Geometry: final body of the model. Coordinates: model frame, mm. A direction names the side the tool comes from. Give positions to 0.01 mm unless a question says otherwise; leave off trailing zeros. Write each loop counter-clockwise with the first axis right and the second up, starting at its lowest first coordinate (ties: lowest second). Pieces come first, ordered by that corner, then holes. Notation, with made-up numbers: (74, 89) -> (133, 89) arc R25 cw to (133, 106) -> close; hole circle Ø5 at (31.25, -37.5). An arc over 180 degrees is marked (long way). Answer as a JSON object with one key per item and string values. Group by question number.
(1) Contact query for flat-ended pins moving along their axis: pin 1 Ø3 at (x, y) = (10, -12.5) entering from +Z; pin 2 Ø5 at (x, z) = (0, 8.5) entering from +Y; pin 3 Ø2 at (x, y) = (12, -38) entering from -Z. Output: stop coordinate, or through.
(2) Set-up query: faces 4 (the face through (-5.89, -30.65, 2.86)), 5 (the face through (-0.28, 38.6, 0.86)), 6 (the face through (16.25, -38.51, 5.96)), 7 (the face through (16.75, -35.53, 6.05)). Return all of +Z, -Z, +X, -X, +Y, -Y with unobstructed straight access to the full face (end or side cutting, diameter ignored); none if empty.
(3) Material intervals for probe 1 along Y at (x, z) = (-10.5, 11.5); probe 2 along X at (y, z) = (3.5, 4.5); probe 3 along X at (y, z) = (9, 11.5), sorted ascending.
(4) Draft query along Z for faces 1 (the face through (24.196, -36.789, 13.507)), 2 (the face through (0.28, -38.6, 0.86)), 3 (the face through (11, -39, 4.25)). Return one class per face: +Z half, -Z half, draft (parallel to the pull), parting line (faces both ways), or undercut.
(5) Section query C-C on y = 27. Output: boundary loops of the cut face in (x, z).
(6) Section query B-B on y = -4.5. Output: boundary loops of the cut face in (x, z).
(7) Section query A-A on x = -10. Output: boundary loops of the cut face in (y, z).
from build123d import *

# Parameters (mm, degrees)
PAD_DEPTH       = 2
PAD001_DEPTH    = 12
FILLET_R        = 3
SKETCH002_R     = 2
POCKET_DEPTH    = 5
POCKET003_DEPTH = 1
SKETCH016_W     = 16
SKETCH016_H     = 2
PAD007_DEPTH    = 10
FILLET002_R     = 3
PAD008_DEPTH    = 4
SKETCH019_R     = 3.25
POCKET005_DEPTH = 2
FILLET004_R     = 1
SKETCH020_W     = 5
SKETCH020_H     = 50
PAD009_DEPTH    = 8
FILLET005_R     = 2
SKETCH021_R     = 3.25
POCKET006_DEPTH = 50


with BuildPart() as part:
    # Sketch → Pad (new body)
    with BuildSketch(Plane.XY):
        with BuildLine():
            Line((-27, 32.5), (-27, -32.5))
            ThreePointArc((-27, -32.5), (-24.949747, -37.449747), (-20, -39.5))
            Line((-20, -39.5), (20, -39.5))
            ThreePointArc((20, -39.5), (24.949747, -37.449747), (27, -32.5))
            Line((27, -32.5), (27, 32.5))
            ThreePointArc((27, 32.5), (24.949747, 37.449747), (20, 39.5))
            Line((20, 39.5), (-20, 39.5))
            ThreePointArc((-20, 39.5), (-24.949747, 37.449747), (-27, 32.5))
        make_face()
    extrude(amount=PAD_DEPTH)

    # Sketch001 (on Face10 of Pad) → Pad001 (join)
    with BuildSketch(Plane.XY.offset(2)):
        with BuildLine():
            Line((-27, 32.5), (-27, -32.5))
            ThreePointArc((-27, -32.5), (-24.949747, -37.449747), (-20, -39.5))
            Line((-20, -39.5), (20, -39.5))
            ThreePointArc((20, -39.5), (24.949747, -37.449747), (27, -32.5))
            Line((27, -32.5), (27, 32.5))
            ThreePointArc((27, 32.5), (24.949747, 37.449747), (20, 39.5))
            Line((20, 39.5), (-20, 39.5))
            ThreePointArc((-20, 39.5), (-24.949747, 37.449747), (-27, 32.5))
        make_face()
        with BuildLine():
            Line((-25, 32.5), (-25, -32.5))
            ThreePointArc((-25, -32.5), (-23.535534, -36.035534), (-20, -37.5))
            Line((-20, -37.5), (20, -37.5))
            ThreePointArc((20, -37.5), (23.535534, -36.035534), (25, -32.5))
            Line((25, -32.5), (25, 32.5))
            ThreePointArc((25, 32.5), (23.535534, 36.035534), (20, 37.5))
            Line((20, 37.5), (-20, 37.5))
            ThreePointArc((-20, 37.5), (-23.535534, 36.035534), (-25, 32.5))
        make_face(mode=Mode.SUBTRACT)
    extrude(amount=PAD001_DEPTH)

    # Fillet
    fillet_edges = [part.edges().sort_by_distance(p)[0] for p in [
        (0, -39.5, 0),
    ]]
    fillet(fillet_edges, radius=FILLET_R)

    # Sketch002 (on Face10 of Fillet) → Pocket (cut)
    with BuildSketch(Plane.XZ.offset(39.5)):
        with Locations((-10, 8.5)):
            Circle(SKETCH002_R)
        with BuildLine():
            ThreePointArc((8.3, 7.75), (6.55, 6), (8.3, 4.25))
            Line((8.3, 4.25), (14.5, 4.25))
            ThreePointArc((14.5, 4.25), (16.25, 6), (14.5, 7.75))
            Line((8.3, 7.75), (14.5, 7.75))
        make_face()
    extrude(amount=-POCKET_DEPTH, mode=Mode.SUBTRACT)

    # Sketch007 → Pocket003 (cut)
    with BuildSketch(Plane.XY.offset(14)):
        with BuildLine():
            Line((-26, 32.5), (-26, -32.5))
            ThreePointArc((-26, -32.5), (-24.242641, -36.742641), (-20, -38.5))
            Line((-20, -38.5), (20, -38.5))
            ThreePointArc((20, -38.5), (24.242641, -36.742641), (26, -32.5))
            Line((26, -32.5), (26, 32.5))
            ThreePointArc((26, 32.5), (24.242641, 36.742641), (20, 38.5))
            Line((20, 38.5), (-20, 38.5))
            ThreePointArc((-20, 38.5), (-24.242641, 36.742641), (-26, 32.5))
        make_face()
        with BuildLine():
            Line((-25, 32.5), (-25, -32.5))
            ThreePointArc((-25, -32.5), (-23.535534, -36.035534), (-20, -37.5))
            Line((-20, -37.5), (20, -37.5))
            ThreePointArc((20, -37.5), (23.535534, -36.035534), (25, -32.5))
            Line((25, -32.5), (25, 32.5))
            ThreePointArc((25, 32.5), (23.535534, 36.035534), (20, 37.5))
            Line((20, 37.5), (-20, 37.5))
            ThreePointArc((-20, 37.5), (-23.535534, 36.035534), (-25, 32.5))
        make_face(mode=Mode.SUBTRACT)
    extrude(amount=-POCKET003_DEPTH, mode=Mode.SUBTRACT)

    # Sketch016 (on Face34 of Pocket003) → Pad007 (join)
    with BuildSketch(Plane.XY.offset(2)):
        with Locations((-6, -32.55)):
            Rectangle(SKETCH016_W, SKETCH016_H)
    extrude(amount=PAD007_DEPTH)

    # Fillet002
    fillet002_edges = [part.edges().sort_by_distance(p)[0] for p in [
        (-6, -31.55, 2),
    ]]
    fillet(fillet002_edges, radius=FILLET002_R)

    # Sketch017 (on Face12 of Fillet002) → Pad008 (join)
    with BuildSketch(Plane(origin=(0, -37.5, 0), x_dir=(-1, 0, 0), z_dir=(0, 1, 0))):
        with BuildLine():
            ThreePointArc((-14.5, 8.25), (-16.75, 6), (-14.5, 3.75))
            Line((-14.5, 3.75), (-8.3, 3.75))
            ThreePointArc((-8.3, 3.75), (-6.05, 6), (-8.3, 8.25))
            Line((-14.5, 8.25), (-8.3, 8.25))
        make_face()
        with BuildLine():
            ThreePointArc((-14.5, 7.85), (-16.35, 6), (-14.5, 4.15))
            Line((-14.5, 4.15), (-8.3, 4.15))
            ThreePointArc((-8.3, 4.15), (-6.45, 6), (-8.3, 7.85))
            Line((-14.5, 7.85), (-8.3, 7.85))
        make_face(mode=Mode.SUBTRACT)
    extrude(amount=PAD008_DEPTH)

    # Sketch019 (on Face46 of Pad008) → Pocket005 (cut)
    with BuildSketch(Plane(origin=(0, 39.5, 0), x_dir=(-1, 0, 0), z_dir=(0, 1, 0))):
        with Locations((0, 8.5)):
            Circle(SKETCH019_R)
    extrude(amount=-POCKET005_DEPTH, mode=Mode.SUBTRACT)

    # Fillet004
    fillet004_edges = [part.edges().sort_by_distance(p)[0] for p in [
        (3.25, 39.5, 8.5),
    ]]
    fillet(fillet004_edges, radius=FILLET004_R)

    # Sketch020 (on Face5 of Fillet004) → Pad009 (join)
    with BuildSketch(Plane.XY.offset(2)):
        Rectangle(SKETCH020_W, SKETCH020_H)
    extrude(amount=PAD009_DEPTH)

    # Fillet005
    fillet005_edges = [part.edges().sort_by_distance(p)[0] for p in [
        (2.5, 0, 2),
        (-2.5, 0, 2),
    ]]
    fillet(fillet005_edges, radius=FILLET005_R)

    # Sketch021 (on Face4 of Fillet005) → Pocket006 (cut)
    with BuildSketch(Plane(origin=(0, 25, 0), x_dir=(-1, 0, 0), z_dir=(0, 1, 0))):
        with Locations((0, 8.5)):
            Circle(SKETCH021_R)
    extrude(amount=-POCKET006_DEPTH, mode=Mode.SUBTRACT)


solid = part.part
Answer list:
{
 "1": {"pin 1": "z = 2", "pin 2": "y = -31.55", "pin 3": "z = 0.04"},
 "2": {"face 4": "+Z", "face 5": "-Z, +X, -X, +Y", "face 6": "-Y", "face 7": "none"},
 "3": {"probe 1": "-39.5 to -37.5, -33.55 to -31.55, 37.5 to 39.5", "probe 2": "-27 to -25, -2.5 to 2.5, 25 to 27", "probe 3": "-27 to -25, 25 to 27"},
 "4": {"face 1": "draft", "face 2": "-Z half", "face 3": "undercut"},
 "5": {"outline": "(-27, 3) arc R3 ccw to (-24, 0) -> (24, 0) arc R3 ccw to (27, 3) -> (27, 14) -> (26, 14) -> (26, 13) -> (25, 13) -> (25, 2) -> (-25, 2) -> (-25, 13) -> (-26, 13) -> (-26, 14) -> (-27, 14) -> close"},
 "6": {"outline": "(-27, 3) arc R3 ccw to (-24, 0) -> (24, 0) arc R3 ccw to (27, 3) -> (27, 14) -> (26, 14) -> (26, 13) -> (25, 13) -> (25, 2) -> (4.5, 2) arc R2 cw to (2.5, 4) -> (2.5, 6.42) arc R3.25 cw to (-2.5, 6.42) -> (-2.5, 4) arc R2 cw to (-4.5, 2) -> (-25, 2) -> (-25, 13) -> (-26, 13) -> (-26, 14) -> (-27, 14) -> close"},
 "7": {"outline": "(-39.5, 3) arc R3 ccw to (-36.5, 0) -> (36.5, 0) arc R3 ccw to (39.5, 3) -> (39.5, 14) -> (38.5, 14) -> (38.5, 13) -> (37.5, 13) -> (37.5, 2) -> (-28.55, 2) arc R3 cw to (-31.55, 5) -> (-31.55, 12) -> (-33.55, 12) -> (-33.55, 2) -> (-37.5, 2) -> (-37.5, 6.5) -> (-39.5, 6.5) -> close; (-39.5, 10.5) -> (-37.5, 10.5) -> (-37.5, 13) -> (-38.5, 13) -> (-38.5, 14) -> (-39.5, 14) -> close"}
}
